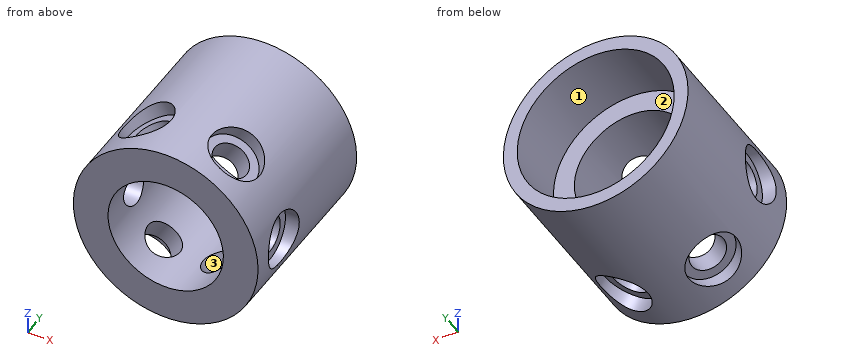
```python
from build123d import *

# Parameters (mm, degrees)
SKETCH1_R           = 20
BOSS_EXTRUDE1_DEPTH = 38
SKETCH2_R           = 12.5
CUT_EXTRUDE1_DEPTH  = 38
SKETCH3_R           = 17
CUT_EXTRUDE2_DEPTH  = 14


with BuildPart() as part:
    # Sketch1 → Boss-Extrude1 (new body)
    with BuildSketch(Plane(origin=(0, 0, 0), x_dir=(1, 0, 0), z_dir=(0, 1, 0))):
        with Locations(Location((0, 0, 0), (0, 0, 270))):
            Circle(SKETCH1_R)
    extrude(amount=BOSS_EXTRUDE1_DEPTH)

    # Sketch2 → Cut-Extrude1 (cut)
    with BuildSketch(Plane(origin=(0, 38, 0), x_dir=(1, 0, 0), z_dir=(0, 1, 0))):
        with Locations(Location((0, 0, 0), (0, 0, 270))):
            Circle(SKETCH2_R)
    extrude(amount=-CUT_EXTRUDE1_DEPTH, mode=Mode.SUBTRACT)

    # Sketch3 → Cut-Extrude2 (cut)
    with BuildSketch(Plane(origin=(0, 38, 0), x_dir=(1, 0, 0), z_dir=(0, 1, 0))):
        with Locations(Location((0, 0, 0), (0, 0, 270))):
            Circle(SKETCH3_R)
    extrude(amount=-CUT_EXTRUDE2_DEPTH, mode=Mode.SUBTRACT)

    # Sketch7 → Cut-Revolve4 (revolve, cut)
    with BuildSketch(Plane.XY, mode=Mode.PRIVATE) as cut_revolve4_sk:
        Polygon((-17, 6), (17, 6), (17, 4), (20, 4), (20, 9.95), (-20, 9.95), (-20, 4), (-17, 4), align=None)
    revolve(cut_revolve4_sk.sketch.rotate(Axis((-20, 9.95, 0), (1, 0, 0)), 270), axis=Axis((-20, 9.95, 0), (1, 0, 0)), mode=Mode.SUBTRACT)

    # Sketch10 → Cut-Revolve5 (revolve, cut)
    with BuildSketch(Plane(origin=(0, 0, 0), x_dir=(-0.5000000000000039, 0, -0.8660254037844365), z_dir=(0.8660254037844364, 0, -0.5000000000000038)), mode=Mode.PRIVATE) as cut_revolve5_sk:
        Polygon((-17, 6), (17, 6), (17, 4), (20, 4), (20, 9.95), (-20, 9.95), (-20, 4), (-17, 4), align=None)
    revolve(cut_revolve5_sk.sketch.rotate(Axis((10, 9.95, 17.320508076), (-0.5000000000000039, 0, -0.8660254037844365)), 270), axis=Axis((10, 9.95, 17.320508076), (-0.5000000000000039, 0, -0.8660254037844365)), mode=Mode.SUBTRACT)

    # Sketch11 → Cut-Revolve6 (revolve, cut)
    with BuildSketch(Plane(origin=(0, 0, 0), x_dir=(0.49999999999999833, 0, -0.8660254037844396), z_dir=(0.8660254037844397, 0, 0.4999999999999984)), mode=Mode.PRIVATE) as cut_revolve6_sk:
        Polygon((-17, 6), (17, 6), (17, 4), (20, 4), (20, 9.95), (-20, 9.95), (-20, 4), (-17, 4), align=None)
    revolve(cut_revolve6_sk.sketch.rotate(Axis((-10, 9.95, 17.320508076), (0.49999999999999833, 0, -0.8660254037844397)), 270), axis=Axis((-10, 9.95, 17.320508076), (0.49999999999999833, 0, -0.8660254037844397)), mode=Mode.SUBTRACT)


solid = part.part
```
For this review, take the finished solid that the model builds, in its own axes (mm). Face numbers are marked on the shaded views. Give positions to 0.01 mm unless a question says otherwise; leave off trailing zeros. Write each loop counter-clockwise with the first axis right and the second up, starting at its lowest first coordinate (ties: lowest second). Pieces come first, ordered by that corner, then holes. Notation, with made-up numbers: M -37.5,13 L 15.5,13 A29 cw 15.5,42 Z; hole C -34,-15.5 d3. An arc over 180 degrees is marked long. Answer as a JSON object with one key per item and string values. Group by question number.
Item 1: Draft analysis for pull direction Y (two halves, no side actions). For the marked faces 1, 2 and 3, state which applies: +Y half, -Y half, draft (parallel to the pull), parting line (faces both ways), or undercut.
Item 2: Consider section D-D on y = 9.95. Count the separate pieces of the cut face and the enclosed holes in it, plus the area to 3 significant figures.
Item 3: Consider section B-B on z = 0.5. Write out the cut boundary in (x, y).
Item 4: Consider section A-A on x = 0. Write out the cut boundary in (y, z), plus the area to 3 significant figures.
Item 5: For probe 1 along X at (y, z) = (34, 0); probe 2 along Y at (x, z) = (-9.5, -16.5); probe 3 along X at (y, z) = (5.5, 0), list the stretches that pass through material, from the lowest coordinate up. Write a range as [from, to].
Item 6: Consider section C-C on z = -4.5. Write out the cut boundary in (x, y), plus the area to 3 significant figures.
Item 7: For pin 1 Ø2 at (x, y) = (3.5, 30) entering from +Z; pin 2 Ø10 at (x, y) = (-9, 27) entering from +Z; pin 3 Ø1.5 at (y, z) = (15, -10) entering from +X; pin 4 Ø15 at (x, z) = (0, 0) entering from -Y, all flat-tipped, find the tip position at first contact; note any pin that passes through.
Check result:
{
 "1": {"face 1": "draft", "face 2": "+Y half", "face 3": "undercut"},
 "2": {"separate pieces": "6", "enclosed holes": "0", "area": "350 mm^2"},
 "3": {"outline": "M -19.99,0 L -12.49,0 L -12.49,6.03 L -17,6.03 L -17,4.02 L -19.99,4.02 Z; M -19.99,15.88 L -17,15.88 L -17,13.87 L -12.49,13.87 L -12.49,24 L -16.99,24 L -16.99,38 L -19.99,38 Z; M 12.49,0 L 19.99,0 L 19.99,4.02 L 17,4.02 L 17,6.03 L 12.49,6.03 Z; M 12.49,13.87 L 17,13.87 L 17,15.88 L 19.99,15.88 L 19.99,38 L 16.99,38 L 16.99,24 L 12.49,24 Z"},
 "4": {"outline": "M 0,-20 L 38,-20 L 38,-17 L 24,-17 L 24,-12.5 L 0,-12.5 Z; M 0,12.5 L 24,12.5 L 24,17 L 38,17 L 38,20 L 0,20 Z", "area": "444 mm^2"},
 "5": {"probe 1": "x = [-20, -17], [17, 20]", "probe 2": "y = [0, 4], [15.9, 38]", "probe 3": "x = [-17, -12.5], [12.5, 17]"},
 "6": {"outline": "M -19.49,0 L -11.66,0 L -11.66,24 L -16.39,24 L -16.39,38 L -19.49,38 L -19.49,13.84 L -17,13.84 L -17,6.06 L -19.49,6.06 Z; M 11.66,0 L 19.49,0 L 19.49,6.06 L 17,6.06 L 17,13.84 L 19.49,13.84 L 19.49,38 L 16.39,38 L 16.39,24 L 11.66,24 Z", "area": "424 mm^2"},
 "7": {"pin 1": "stops at z = 19.84", "pin 2": "stops at z = 19.6", "pin 3": "stops at x = 17.73", "pin 4": "passes through"}
}
